Build history of the part. All positions in model axes, mm. Face numbers are marked on the shaded views. A direction names the side the tool comes from. Round coordinates to 2 decimals unless told otherwise and drop trailing zeros. Write each loop counter-clockwise with the first axis right and the second up, starting at its lowest first coordinate (ties: lowest second). Pieces come first, ordered by that corner, then holes. Notation, with made-up numbers: (25.25, 88) -> (73.25, 88) arc R16 ccw to (73.25, 96) -> close; hole circle Ø2 at (-5, 60). An arc over 180 degrees is marked (long way). Answer in a Markdown table with one row per item.
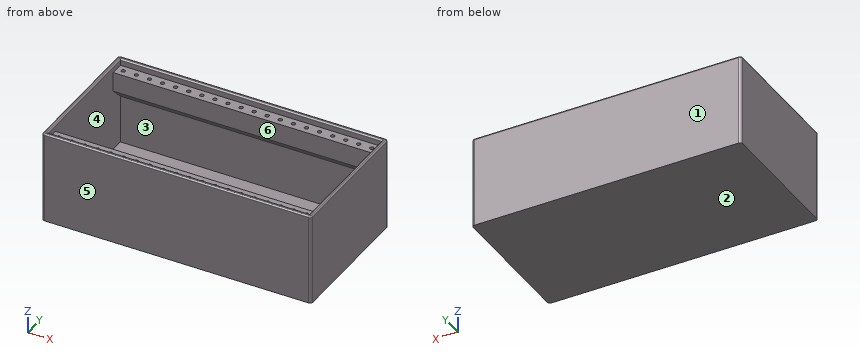
Autodesk Fusion 360 part; units mm, degrees
sketch "Sketch1" plane through (0, 0, 0) normal (0, 0, 1) x (1, 0, 0)
  line L0 (0, 0) -> (200, 0)
  line L1 (200, 0) -> (200, 100)
  line L2 (200, 100) -> (0, 100)
  line L3 (0, 100) -> (0, 0)
  line L4 (-3, -3) -> (203, -3)
  line L5 (203, -3) -> (203, 103)
  line L6 (203, 103) -> (-3, 103)
  line L7 (-3, 103) -> (-3, -3)
  line L8 (0, 100) -> (0, 103)
  line L9 (0, 0) -> (0, -3)
  line L10 (200, 0) -> (200, -3)
  line L11 (200, 100) -> (200, 103)
  circle A0 centre (5, 95) radius 1.5
  line L12 (0, 90) -> (200, 90)
  line L13 (0, 10) -> (200, 10)
  circle A1 centre (15, 95) radius 1.5
  circle A2 centre (25, 95) radius 1.5
  circle A3 centre (35, 95) radius 1.5
  circle A4 centre (45, 95) radius 1.5
  circle A5 centre (55, 95) radius 1.5
  circle A6 centre (65, 95) radius 1.5
  circle A7 centre (75, 95) radius 1.5
  circle A8 centre (85, 95) radius 1.5
  circle A9 centre (95, 95) radius 1.5
  circle A10 centre (105, 95) radius 1.5
  circle A11 centre (115, 95) radius 1.5
  circle A12 centre (125, 95) radius 1.5
  circle A13 centre (135, 95) radius 1.5
  circle A14 centre (145, 95) radius 1.5
  circle A15 centre (5, 5) radius 1.5
  circle A16 centre (15, 5) radius 1.5
  circle A17 centre (25, 5) radius 1.5
  circle A18 centre (35, 5) radius 1.5
  circle A19 centre (45, 5) radius 1.5
  circle A20 centre (55, 5) radius 1.5
  circle A21 centre (65, 5) radius 1.5
  circle A22 centre (75, 5) radius 1.5
  circle A23 centre (85, 5) radius 1.5
  circle A24 centre (95, 5) radius 1.5
  circle A25 centre (105, 5) radius 1.5
  circle A26 centre (115, 5) radius 1.5
  circle A27 centre (125, 5) radius 1.5
  circle A28 centre (135, 5) radius 1.5
  circle A29 centre (145, 5) radius 1.5
  circle A30 centre (155, 95) radius 1.5
  circle A31 centre (165, 95) radius 1.5
  circle A32 centre (175, 95) radius 1.5
  circle A33 centre (185, 95) radius 1.5
  circle A34 centre (195, 95) radius 1.5
  circle A35 centre (155, 5) radius 1.5
  circle A36 centre (165, 5) radius 1.5
  circle A37 centre (175, 5) radius 1.5
  circle A38 centre (185, 5) radius 1.5
  circle A39 centre (195, 5) radius 1.5
  dimension "d1" = 3
  dimension "d2" = 3
  dimension "d5" = 190
  dimension "d6" = -90
  dimension "d23" = 200
  dimension "d33" = 100
extrude "Extrude1" add sketch "Sketch1" along normal blind 15 from surface at 50 contours L0 L1 L3 L13 | L3 L4 L6 L7 L8 L9 | L0 L4 L9 L10 | L1 L4 L5 L6 L10 L11 | L1 L2 L3 L12 | L2 L6 L8 L11 makes body 1
extrude "Extrude2" add sketch "Sketch1" along normal blind 3 separate body contours L0 L1 L3 L13 | L3 L4 L6 L7 L8 L9 | L0 L4 L9 L10 | L1 L4 L5 L6 L10 L11 | L1 L3 L12 L13 | L1 L2 L3 L12 | L2 L6 L8 L11 | A0 | A1 | A2 | A3 | A4 | A5 | A6 | A7 | A8 | A9 | A10 | A11 | A12 | A13 | A14 | A15 | A16 | A17 | A18 | A19 | A20 | A21 | A22 | A23 | A24 | A25 | A26 | A27 | A28 | A29 | A30 | A31 | A32 | A33 | A34 | A35 | A36 | A37 | A38 | A39 makes body 2
extrude "Extrude3" add sketch "Sketch1" along normal blind 50 contours L3 L4 L6 L7 L8 L9 | L0 L4 L9 L10 | L1 L4 L5 L6 L10 L11 | L2 L6 L8 L11 bodies 1 2
sketch "Sketch2" plane through (0, 0, 0) normal (1, 0, 0) x (0, 1, 0)
  line L0 (90, 50) -> (90, 65)
  line L1 (90, 65) -> (10, 65)
  line L2 (10, 65) -> (10, 50)
  line L3 (10, 50) -> (0, 50)
  line L4 (0, 50) -> (0, 3)
  line L5 (0, 3) -> (100, 3)
  line L6 (100, 3) -> (100, 50)
  line L7 (100, 50) -> (90, 50)
  line L8 (90, 50) -> (100, 40)
  line L9 (10, 50) -> (0, 40)
  line L10 (103, 0) -> (-3, 0)
  dimension "d34" = 40
extrude "Extrude4" add sketch "Sketch2" along normal up to surface (200 mm away) contours L6 L7 L8 | L3 L4 L9 bodies 1
extrude "Extrude5" add sketch "Sketch1" along normal blind 5 from surface at 65 contours L3 L4 L6 L7 L8 L9 | L0 L4 L9 L10 | L1 L4 L5 L6 L10 L11 | L2 L6 L8 L11 bodies 1
fillet "Fillet1" radius 2 4 edges at (-3, -3, 35) (203, 103, 35) (203, -3, 35) (-3, 103, 35) on bodies 1
fillet "Fillet2" radius 1 12 edges at (-2.4142, 102.4142, 70) (-3, 50, 70) (-2.4142, -2.4142, 70) (100, -3, 70) (202.4142, -2.4142, 70) (203, 50, 70) (202.4142, 102.4142, 70) (100, 103, 70) (100, 100, 70) (0, 50, 70) (100, 0, 70) (200, 50, 70) on bodies 1
equation "d7 = depth - 20 mm"
equation "d12 = depth - 20 mm"
equation "d16 = depth - 5 mm"
equation "d23 = width"
equation "width = ( userWidth * 1 ) * 1 mm"
equation "depth = ( userDepth * 1 ) * 1 mm"
equation "height = ( userHeight * 1 ) * 1 mm"
equation "d34 = depth - 30 mm"
Q1. Wall check: line 1 (Y direction, x = 75, z = 60.5); line 2 (X direction, y = 75, z = 20); line 3 (Y direction, x = 107, z = 52). Give the ranges that are in metal, low to high. Write a range as [from, to].
A:
| item | result |
|---|---|
| line 1 | [-3, 3.5], [6.5, 10], [90, 93.5], [96.5, 103] |
| line 2 | [-3, 0], [200, 203] |
| line 3 | [-3, 10], [90, 103] |
Q2. Saw through at A-A on z = 45. Write the cut outline in (x, y).
A:
| item | result |
|---|---|
| outline | (-3, -1) arc R2 ccw to (-1, -3) -> (201, -3) arc R2 ccw to (203, -1) -> (203, 101) arc R2 ccw to (201, 103) -> (-1, 103) arc R2 ccw to (-3, 101) -> close; hole (0, 5) -> (200, 5) -> (200, 95) -> (0, 95) -> close |
Q3. Saw through at C-C on y = 83.5. Write the cut outline in (x, z).
A:
| item | result |
|---|---|
| outline | (-3, 0) -> (203, 0) -> (203, 69) arc R1 ccw to (202, 70) -> (201, 70) arc R1 ccw to (200, 69) -> (200, 3) -> (0, 3) -> (0, 69) arc R1 ccw to (-1, 70) -> (-2, 70) arc R1 ccw to (-3, 69) -> close |
Q4. Saw through at D-D on z = 14.5. Write the cut outline in (x, y).
A:
| item | result |
|---|---|
| outline | (-3, -1) arc R2 ccw to (-1, -3) -> (201, -3) arc R2 ccw to (203, -1) -> (203, 101) arc R2 ccw to (201, 103) -> (-1, 103) arc R2 ccw to (-3, 101) -> close; hole (0, 0) -> (200, 0) -> (200, 100) -> (0, 100) -> close |
Q5. Which spindle directions (+Z, -Z, +X, -X, +Y, -Y) get a long thin tool onto all of the face, cutting with end or side? Do the marked faces 4, 5 and 6. Say none if no direction does.
A:
| item | result |
|---|---|
| face 4 | none |
| face 5 | +Z, -Z, +X, -X, -Y |
| face 6 | +Z |
Q6. Saw through at B-B on x = 111. Write the cut outline in (y, z), plus the area to 3 significant figures.
A:
| item | result |
|---|---|
| outline | (-3, 0) -> (103, 0) -> (103, 69) arc R1 ccw to (102, 70) -> (101, 70) arc R1 ccw to (100, 69) -> (100, 65) -> (90, 65) -> (90, 50) -> (100, 40) -> (100, 3) -> (0, 3) -> (0, 40) -> (10, 50) -> (10, 65) -> (0, 65) -> (0, 69) arc R1 ccw to (-1, 70) -> (-2, 70) arc R1 ccw to (-3, 69) -> close |
| area | 1,120 mm² |
Q7. Two-plate mould, pull along Y, no slides. Class the marked faces 1, 2 and 3: released by +Y, released by -Y, zero draft, split by the parting line, or undercut.
A:
| item | result |
|---|---|
| face 1 | released by +Y |
| face 2 | zero draft |
| face 3 | undercut |
Q8. Drop flat-ended pins along their axis: P1, Ø2, axis at x = 27, y = 38.5, coming from the +Z side; P2, Ø5, axis at x = 115, y = 95, coming from the +Z side; P3, Ø0.9, axis at x = 125, y = 94.5, coming from the +Z side. Give the stop position or say it passes through.
A:
| item | result |
|---|---|
| P1 | z = 3 |
| P2 | z = 65 |
| P3 | z = 50 |
